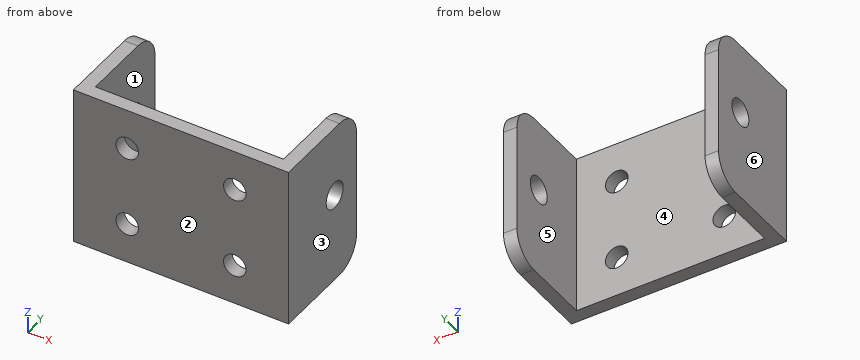
from build123d import *

# Parameters (mm, degrees)
BOSS_EXTRUDE1_DEPTH = 38.1
SKETCH2_R           = 3.175
CUT_EXTRUDE1_DEPTH  = 65.757547823
CUT_EXTRUDE2_REACH  = 52.899
SKETCH3_R           = 2.667
FILLET1_R           = 6.35


with BuildPart() as part:
    # Sketch1 → Boss-Extrude1 (new body)
    with BuildSketch(Plane.XY):
        Polygon((-22.225, -9.525), (-22.225, 12.7), (-25.4, 12.7), (-25.4, -12.7), (25.4, -12.7), (25.4, 12.7), (22.225, 12.7), (22.225, -9.525), align=None)
    extrude(amount=BOSS_EXTRUDE1_DEPTH)

    # Sketch2 → Cut-Extrude1 (cut, through all)
    with BuildSketch(Plane.ZY.offset(25.4)):
        with Locations((21.233208268, 4.543167929)):
            Circle(SKETCH2_R)
    extrude(amount=-CUT_EXTRUDE1_DEPTH, mode=Mode.SUBTRACT)

    # Sketch3 → Cut-Extrude2 (cut, up to next)
    with BuildSketch(Plane(origin=(0, -9.525, 0), x_dir=(1, 0, 0), z_dir=(0, 1, 0)), mode=Mode.PRIVATE) as cut_extrude2_sk1:
        with Locations(Location((12.7, -9.525, 0), (0, 0, 270))):
            Circle(SKETCH3_R)
    cut_extrude2_tool1 = extrude(cut_extrude2_sk1.sketch, amount=-CUT_EXTRUDE2_REACH, mode=Mode.PRIVATE) & part.part
    # Sketch3 → Cut-Extrude2 (cut, up to next)
    with BuildSketch(Plane(origin=(0, -9.525, 0), x_dir=(1, 0, 0), z_dir=(0, 1, 0)), mode=Mode.PRIVATE) as cut_extrude2_sk2:
        with Locations(Location((12.7, -28.575, 0), (0, 0, 270))):
            Circle(SKETCH3_R)
    cut_extrude2_tool2 = extrude(cut_extrude2_sk2.sketch, amount=-CUT_EXTRUDE2_REACH, mode=Mode.PRIVATE) & part.part
    # Sketch3 → Cut-Extrude2 (cut, up to next)
    with BuildSketch(Plane(origin=(0, -9.525, 0), x_dir=(1, 0, 0), z_dir=(0, 1, 0)), mode=Mode.PRIVATE) as cut_extrude2_sk3:
        with Locations(Location((-12.7, -28.575, 0), (0, 0, 270))):
            Circle(SKETCH3_R)
    cut_extrude2_tool3 = extrude(cut_extrude2_sk3.sketch, amount=-CUT_EXTRUDE2_REACH, mode=Mode.PRIVATE) & part.part
    # Sketch3 → Cut-Extrude2 (cut, up to next)
    with BuildSketch(Plane(origin=(0, -9.525, 0), x_dir=(1, 0, 0), z_dir=(0, 1, 0)), mode=Mode.PRIVATE) as cut_extrude2_sk4:
        with Locations(Location((-12.7, -9.525, 0), (0, 0, 270))):
            Circle(SKETCH3_R)
    cut_extrude2_tool4 = extrude(cut_extrude2_sk4.sketch, amount=-CUT_EXTRUDE2_REACH, mode=Mode.PRIVATE) & part.part
    add(cut_extrude2_tool1.solids().sort_by_distance((12.7, -9.525, 9.525))[0], mode=Mode.SUBTRACT)
    add(cut_extrude2_tool2.solids().sort_by_distance((12.7, -9.525, 28.575))[0], mode=Mode.SUBTRACT)
    add(cut_extrude2_tool3.solids().sort_by_distance((-12.7, -9.525, 28.575))[0], mode=Mode.SUBTRACT)
    add(cut_extrude2_tool4.solids().sort_by_distance((-12.7, -9.525, 9.525))[0], mode=Mode.SUBTRACT)

    # Fillet1
    fillet1_edges = [part.edges().sort_by_distance(p)[0] for p in [
        (-23.8125, 12.7, 38.1),
        (23.8125, 12.7, 38.1),
        (23.8125, 12.7, 0),
        (-23.8125, 12.7, 0),
    ]]
    fillet(fillet1_edges, radius=FILLET1_R)


solid = part.part
Geometry: final body of the model. Coordinates: model frame, mm. Face numbers are marked on the shaded views. A direction names the side the tool comes from. Coordinates: 2 decimals unless noted, no trailing zeros. Loops run counter-clockwise (first coordinate to the right, second up) from the corner with the lowest first, then second, coordinate; pieces in that order, holes last. Notation, with made-up numbers: M -26,23.25 L 17,23.25 A17 ccw 17,47.25 Z; hole C -33.5,5 d11. An arc over 180 degrees is marked long. One line per item, written item: value. Start each with the question number.
1) Pin query (flat end, axial travel): P1, Ø6, axis at x = -12.7, z = 9.525, coming from the +Y side (3 decimals); P2, Ø3, axis at x = 12.7, z = 28.575, coming from the +Y side. Return the tip coordinate at first contact, or that it passes through.
2) Cut plane D-D (z = 28.5). Return loops of the section in (x, y) (3 decimals), then the cut area to 3 significant figures.
3) Cut plane A-A (y = -10.25). Return loops of the section in (x, z) (3 decimals), then the cut area to 3 significant figures.
4) Reachability of the marked faces 5 and 6 from +Z, -Z, +X, -X, +Y, -Y: full face, straight path, thin tool, end or side. Return the list, or none.
5) Material intervals for L1, parallel to X at y = -0.5, z = 24 (3 decimals); L2, parallel to Y at x = -22, z = 23 (3 decimals); L3, parallel to Y at x = 23, z = 32.5, sorted ascending. Write a range as from..to.
6) Cut plane B-B (x = -12.7). Return loops of the section in (y, z) (3 decimals).
7) Cut plane C-C (y = -6). Return loops of the section in (x, z) (3 decimals).
8) Draft query along X for the marked faces 1, 2, 3 and 4. Return one class per face: released by +X, released by -X, zero draft, split by the parting line, or undercut.
Evaluation:
1. P1: y = -9.525
1. P2: through
2. outline: M -25.4,-12.7 L -15.366,-12.7 L -15.366,-9.525 L -22.225,-9.525 L -22.225,12.7 L -25.4,12.7 Z; M -10.034,-12.7 L 10.034,-12.7 L 10.034,-9.525 L -10.034,-9.525 Z; M 15.366,-12.7 L 25.4,-12.7 L 25.4,12.7 L 22.225,12.7 L 22.225,-9.525 L 15.366,-9.525 Z
2. area: 269 mm^2
3. outline: M -25.4,0 L 25.4,0 L 25.4,38.1 L -25.4,38.1 Z; hole C -12.7,9.525 d5.334; hole C -12.7,28.575 d5.334; hole C 12.7,9.525 d5.334; hole C 12.7,28.575 d5.334
3. area: 1,850 mm^2
4. face 5: +Z, -Z, +Y
4. face 6: +Z, -Z, -X, +Y, -Y
5. L1: -25.4..-22.225, 22.225..25.4
5. L2: -12.7..-9.525
5. L3: -12.7..12.66
6. outline: M -12.7,0 L -9.525,0 L -9.525,6.858 L -12.7,6.858 Z; M -12.7,12.192 L -9.525,12.192 L -9.525,25.908 L -12.7,25.908 Z; M -12.7,31.242 L -9.525,31.242 L -9.525,38.1 L -12.7,38.1 Z
7. outline: M -25.4,0 L -22.225,0 L -22.225,38.1 L -25.4,38.1 Z; M 22.225,0 L 25.4,0 L 25.4,38.1 L 22.225,38.1 Z
8. face 1: undercut
8. face 2: zero draft
8. face 3: released by +X
8. face 4: undercut
